from build123d import *

# Parameters (mm, degrees)
SKETCH135_W             = 20
SKETCH135_H             = 42.5
SKETCH135_W_2           = 14
SKETCH135_H_2           = 36.5
CHAMFER006_SIZE         = 4
PAD037_DEPTH            = 20
PAD038_DEPTH            = 3
SKETCH150_W             = 5.2
SKETCH150_H             = 4.25
POCKET048_DEPTH         = 45.001
PAD039_DEPTH            = 42.5
BODY012_ROLL_ANGLE      = 90
BODY012_PLACEMENT_ANGLE = -90


with BuildPart() as part:
    # AdditivePipe002: sweep along a path in Sketch134
    with BuildLine(Plane.XY) as additivepipe002_path:
        Line((0, 0), (0, 260))
    # Sketch135 → AdditivePipe002 (sweep)
    with BuildSketch(Plane.XZ):
        Rectangle(SKETCH135_W, SKETCH135_H)
        Rectangle(SKETCH135_W_2, SKETCH135_H_2, mode=Mode.SUBTRACT)
    sweep(path=additivepipe002_path.line)

    # Chamfer006
    chamfer006_edges = [part.edges().sort_by_distance(p)[0] for p in [
        (10, 130, 21.25),
        (10, 130, -21.25),
        (7, 130, 18.25),
        (7, 130, -18.25),
    ]]
    chamfer(chamfer006_edges, length=CHAMFER006_SIZE)

    # Sketch147 (on Face1 of AdditivePipe002) → Pad037 (new body)
    with BuildSketch(Plane.XZ):
        Polygon((-4.767949, 21.25), (4.797949, 21.25), (6.53, 18.25), (-6.5, 18.25), align=None)
    pad037 = extrude(amount=PAD037_DEPTH)

    # Sketch148 (on Face13 of Pad037) → Pad038 (join, symmetric)
    with BuildSketch(Plane(origin=(0, 0, 0), x_dir=(0, 0, 1), z_dir=(1, 0, 0))):
        Polygon((21.25, 20), (23.75, 17.7), (23.75, 15.2), (21.25, 15.2), align=None)
    pad038 = extrude(amount=PAD038_DEPTH, both=True)

    # Mirrored011: Pad038, Pad037 across Sketch148 V_Axis
    add(pad038.mirror(Plane.XY))
    add(pad037.mirror(Plane.XY))

    # Sketch150 (on Face6 of Chamfer006) → Pocket048 (cut, through all)
    with BuildSketch(Plane(origin=(0, 0, 21.25), x_dir=(-1, 0, 0), z_dir=(0, 0, 1))):
        with Locations((2, -246.975)):
            Rectangle(SKETCH150_W, SKETCH150_H)
    extrude(amount=-POCKET048_DEPTH, mode=Mode.SUBTRACT)

    # Sketch151 (on Face3 of Pocket048) → Pad039 (join)
    with BuildSketch(Plane(origin=(0, 0, -21.25), x_dir=(1, 0, 0), z_dir=(0, 0, -1))):
        Polygon((-20, 0), (-10, 0), (-10, -25), align=None)
    extrude(amount=-PAD039_DEPTH)


with BuildPart() as part_1:
    # Body012 roll: moved
    add(part.part.rotate(Axis((0, 0, 0), (1, 0, 0)), BODY012_ROLL_ANGLE))


with BuildPart() as part_2:
    # Body012 placement: moved
    add(part_1.part.moved(Location((-357.518507, -26.157783, -137.100044))).rotate(Axis((-357.518507, -26.157783, -137.100044), (0, 0, 1)), BODY012_PLACEMENT_ANGLE))


solid = part_2.part
Design review of the part built by this model. Coordinates are the model's own, in mm. A direction names the side the tool comes from. Coordinates: 2 decimals unless noted, no trailing zeros. Loops run counter-clockwise (first coordinate to the right, second up) from the corner with the lowest first, then second, coordinate; pieces in that order, holes last. Notation, with made-up numbers: M -10,76 L 38,76 A15 cw 38,99 Z; hole C 50,53 d5. An arc over 180 degrees is marked long. Use one line per item in the form item = value.
(1) For line 1 along X through (y, z) = (-25.5, 76); line 2 along Y through (x, z) = (-358.5, 53); line 3 along Z through (x, y) = (-355.5, -33.5), list the stretches that pass through material, from the lowest coordinate up. Write a range as from..to.
Return value:
line_1 = -378.77..-375.77, -339.27..-336.27
line_2 = -36.16..-33.16, -19.16..-16.16
line_3 = -137.1..122.9
(2) For faces 3 (the face through (-358, -16.158, 7)), 4 (the face through (-358, -17, 122.9)), 5 (the face through (-357, -19.158, -5)), list the 3-axis set-ups (+Z, -Z, +X, -X, +Y, -Y) from which the entire face can be reached by the end or side of a thin tool; tool diameter is ignored.
Return value:
face_3 = +Z, +X, -X, +Y
face_4 = +Z, +X, -X, +Y, -Y
face_5 = +Z, -Z
(3) Consider section A-A (x = -353). Write out the cut boundary in (y, z), and give its area (4 significant figures).
Return value:
outline = M -36.16,-137.1 L -33.16,-137.1 L -33.16,122.9 L -36.16,122.9 Z; M -19.16,-137.1 L -6.16,-137.1 L -16.16,-112.1 L -16.16,122.9 L -19.16,122.9 Z
area = 1,685 mm2
(4) Consider section B-B (z = 5). Write out the cut boundary in (x, y).
Return value:
outline = M -378.77,-32.16 L -374.77,-36.16 L -340.27,-36.16 L -336.27,-32.16 L -336.27,-16.16 L -378.77,-16.16 Z; hole M -375.77,-29.16 L -371.77,-33.16 L -343.27,-33.16 L -339.27,-29.16 L -339.27,-19.16 L -375.77,-19.16 Z
(5) Consider section C-C (y = -9.5). Write out the cut boundary in (x, z), and give its area (3 significant figures).
Return value:
outline = M -378.77,-137.1 L -336.27,-137.1 L -336.27,-128.74 L -378.77,-128.74 Z
area = 355 mm2
(6) Draft analysis for pull direction X (two halves, no side actions). For faces 1 (the face through (-358, -33.158, -5)), 2 (the face through (-357, -36.158, -5)), state which applies: pulls with the +X half, pulls with the -X half, needs draft (parallel to the pull), parting line crosses it, or undercut.
Return value:
face_1 = undercut
face_2 = needs draft
(7) Clearance check with flat-ended pins moving along their axes: P1, Ø2.5, axis at x = -378, z = 109, coming from the -Y side; P2, Ø1.2, axis at x = -379.5, z = -155.5, coming from the +Y side; P3, Ø8, axis at y = -24.5, z = -63, coming from the -X side. State where each tip first meets the part, or that it passes through.
Return value:
P1 = -34.18
P2 = -23.16
P3 = -378.77
